from build123d import *

# Parameters (mm, degrees)
SKETCH1_W           = 3.175
SKETCH1_H           = 6.35
SKETCH1_W_2         = 19.05
SKETCH1_H_2         = 9.525
SKETCH1_R           = 2.38125
BOSS_EXTRUDE1_DEPTH = 3.175


with BuildPart() as part:
    # Sketch1 → Boss-Extrude1 (new body)
    # profile 1 of 3: a face of its own
    with BuildSketch(Plane.XY):
        with Locations((-11.1125, 0)):
            Rectangle(SKETCH1_W, SKETCH1_H)
    # profile 2 of 3: a face of its own
    with BuildSketch(Plane.XY):
        Rectangle(SKETCH1_W_2, SKETCH1_H_2)
        Circle(SKETCH1_R, mode=Mode.SUBTRACT)
    # profile 3 of 3: a face of its own
    with BuildSketch(Plane.XY):
        with Locations((11.1125, 0)):
            Rectangle(SKETCH1_W, SKETCH1_H)
    extrude(amount=BOSS_EXTRUDE1_DEPTH)


solid = part.part
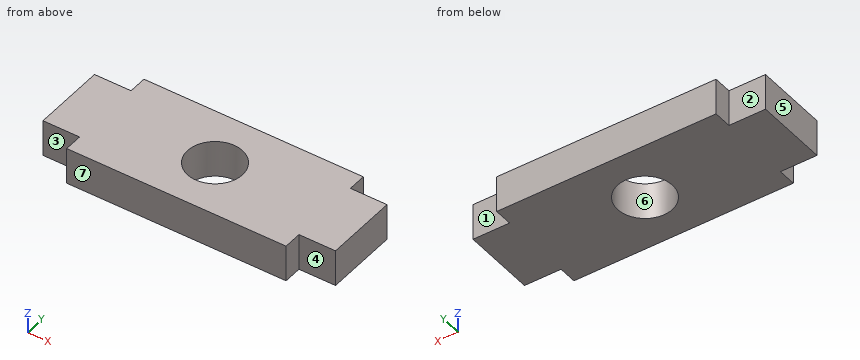
Input: part model. Units: mm. Frame: model coordinates. Face numbers are marked on the shaded views. A direction names the side the tool comes from. Coordinates: 2 decimals unless noted, no trailing zeros. Loops run counter-clockwise (first coordinate to the right, second up) from the corner with the lowest first, then second, coordinate; pieces in that order, holes last. Notation, with made-up numbers: (72.5, 3) -> (104.5, 3) arc R6 ccw to (104.5, 7) -> close; hole circle Ø11 at (-17, -5). An arc over 180 degrees is marked (long way). Write each question's results on one line, items separated by ' | '. Start each with the question number.
Q1. Ray query, line 1 (Y direction, x = 0, z = 1.3); line 2 (Y direction, x = 9.75, z = 1.6) (3 decimals); line 3 (Y direction, x = -2, z = 1.05). Return the intervals inside material, ascending. Write a range as from..to.
Q2. Section A-A, the plane z = 1.8. Return the cut outline in (x, y) (1 decimal).
Q3. Section B-B, the plane x = 0. Return the cut outline in (y, z) (1 decimal), plus the area to 3 significant figures.
Q4. Pull-direction query (Y, two-part tool) for the marked faces 5, 6 and 7; classes: released by +Y, released by -Y, zero draft, split by the parting line, or undercut.
Q5. Section C-C, the plane y = 0. Return the cut outline in (x, z) (3 decimals), plus the area to 3 significant figures.
Q6. Reachability of the marked faces 1, 2, 3 and 4 from +Z, -Z, +X, -X, +Y, -Y: full face, straight path, thin tool, end or side. Return the list, or none.
Q7. Section D-D, the plane y = -4. Return the cut outline in (x, z) (3 decimals), plus the area to 3 significant figures.
Q8. Pin query (flat end, axial travel): pin 1 (1.3 mm diameter, centred on y = 4, z = 1, fed in from +X) (3 decimals); pin 2 (1.3 mm diameter, centred on y = 4, z = 1, fed in from -X) (3 decimals); pin 3 (1 mm diameter, centred on x = 10.5, z = 1.5, fed in from +Y) (3 decimals). Return the tip coordinate at first contact, or that it passes through.
Found:
1) line 1: -4.76..-2.38, 2.38..4.76 | line 2: -3.175..3.175 | line 3: -4.76..-1.29, 1.29..4.76
2) outline: (-12.7, -3.2) -> (-9.5, -3.2) -> (-9.5, -4.8) -> (9.5, -4.8) -> (9.5, -3.2) -> (12.7, -3.2) -> (12.7, 3.2) -> (9.5, 3.2) -> (9.5, 4.8) -> (-9.5, 4.8) -> (-9.5, 3.2) -> (-12.7, 3.2) -> close; hole circle Ø4.8 at (0, 0)
3) outline: (-4.8, 0) -> (-2.4, 0) -> (-2.4, 3.2) -> (-4.8, 3.2) -> close; (2.4, 0) -> (4.8, 0) -> (4.8, 3.2) -> (2.4, 3.2) -> close | area: 15.1 mm2
4) face 5: zero draft | face 6: undercut | face 7: released by -Y
5) outline: (-12.7, 0) -> (-2.381, 0) -> (-2.381, 3.175) -> (-12.7, 3.175) -> close; (2.381, 0) -> (12.7, 0) -> (12.7, 3.175) -> (2.381, 3.175) -> close | area: 65.5 mm2
6) face 1: +Z, -Z, +X, +Y | face 2: +Z, -Z, -X, +Y | face 3: +Z, -Z, -X, -Y | face 4: +Z, -Z, +X, -Y
7) outline: (-9.525, 0) -> (9.525, 0) -> (9.525, 3.175) -> (-9.525, 3.175) -> close | area: 60.5 mm2
8) pin 1: x = 9.525 | pin 2: x = -9.525 | pin 3: y = 3.175
